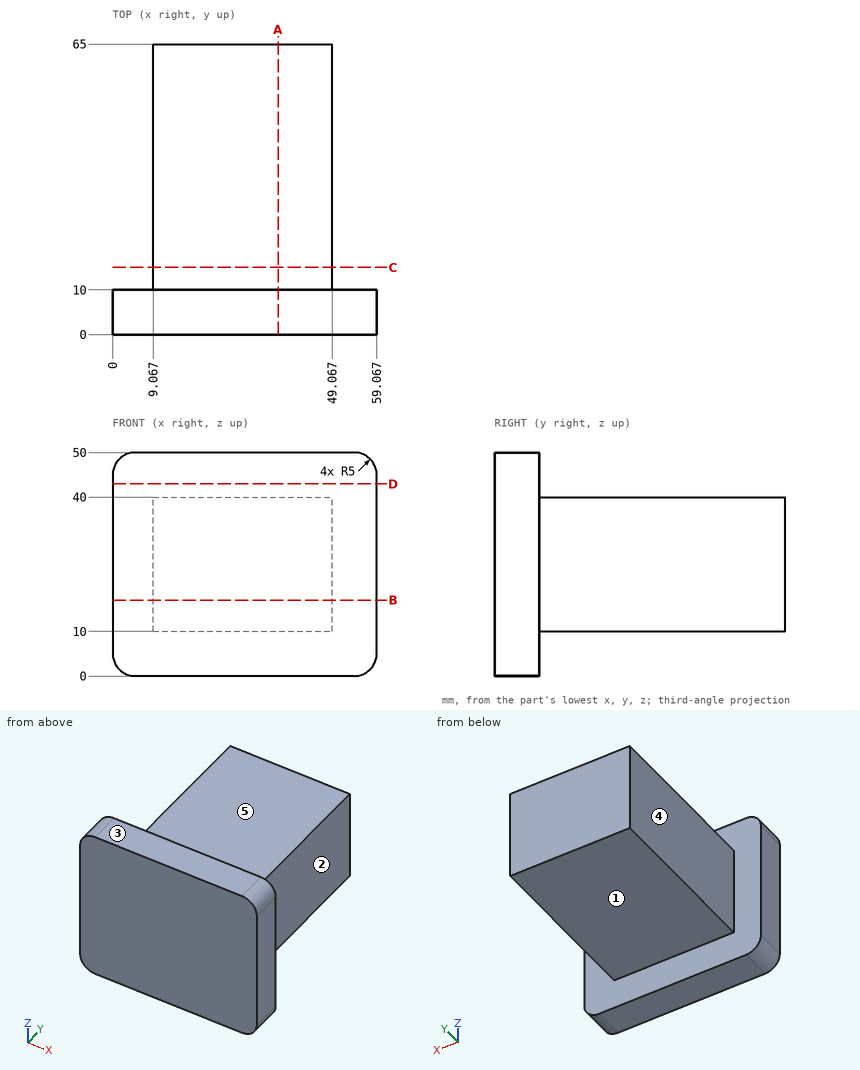
Can you work these out from the drawing? Everything is in mm from the part's minimum corner. A direction names the side the tool comes from. Coordinates: 2 decimals unless noted, no trailing zeros. Loops run counter-clockwise (first coordinate to the right, second up) from the corner with the lowest first, then second, coordinate; pieces in that order, holes last. Notation, with made-up numbers: (5.25, -36.75) - (38.25, -36.75) arc R20 ccw to (38.25, -8.75) - close; hole circle Ø2 at (47.25, 13.5). An arc over 180 degrees is marked (long way). Use a Markdown table: item, result.
Item 1: I want a section at D-D on z = 43. Please give me the cut outline in (x, y), and give its area (3 significant figures).
Numbers:
| item | result |
|---|---|
| outline | (0, 0) - (59.07, 0) - (59.07, 10) - (0, 10) - close |
| area | 591 mm2 |
Item 2: I want a section at A-A on x = 37. Please give me the cut outline in (y, z).
Numbers:
| item | result |
|---|---|
| outline | (0, 0) - (10, 0) - (10, 10) - (65, 10) - (65, 40) - (10, 40) - (10, 50) - (0, 50) - close |
Item 3: I want a section at B-B on z = 17. Please give me the cut outline in (x, y), and give its area (3 significant figures).
Numbers:
| item | result |
|---|---|
| outline | (0, 0) - (59.07, 0) - (59.07, 10) - (49.07, 10) - (49.07, 65) - (9.07, 65) - (9.07, 10) - (0, 10) - close |
| area | 2,790 mm2 |
Item 4: If I drill on probe 1 along Y at (x, z) = (51, 15); probe 2 along Z at (x, y) = (37, 55); probe 3 along X at (y, z) = (15, 24), over which ranges is the centre line in solid material (lowest first)? Write a range as from..to.
Numbers:
| item | result |
|---|---|
| probe 1 | y = 0..10 |
| probe 2 | z = 10..40 |
| probe 3 | x = 9.07..49.07 |
Item 5: For the marked faces 1, 2, 3, 4 and 5, which set-ups out of +Z, -Z, +X, -X, +Y, -Y let a thin tool reach every point of the face, with its end or its side?
Numbers:
| item | result |
|---|---|
| face 1 | -Z, +X, -X, +Y |
| face 2 | +Z, -Z, +X, +Y |
| face 3 | +Z, +X, -X, +Y, -Y |
| face 4 | +Z, -Z, -X, +Y |
| face 5 | +Z, +X, -X, +Y |
Item 6: I want a section at C-C on y = 15. Please give me the cut outline in (x, z).
Numbers:
| item | result |
|---|---|
| outline | (9.07, 10) - (49.07, 10) - (49.07, 40) - (9.07, 40) - close |
Item 7: Will these pins go through, and if not, where does the flat tip stop? pin 1 (1 mm diameter, centred on x = 49.5, z = 11, fed in from -Y); pin 2 (6 mm diameter, centred on x = 47, z = 45, fed in from +Y); pin 3 (2 mm diameter, centred on x = 39.5, y = 33.5, fed in from -Z); pin 4 (15 mm diameter, centred on y = 48.5, z = 21, fed in from -X).
Numbers:
| item | result |
|---|---|
| pin 1 | stops at y = 0 |
| pin 2 | stops at y = 10 |
| pin 3 | stops at z = 10 |
| pin 4 | stops at x = 9.07 |
